Check sheet for the modelled part. Datum: model origin and axes. Units: mm. A direction names the side the tool comes from. Round coordinates to 2 decimals unless told otherwise and drop trailing zeros. Write each loop counter-clockwise with the first axis right and the second up, starting at its lowest first coordinate (ties: lowest second). Pieces come first, ordered by that corner, then holes. Notation, with made-up numbers: M -25.75,-33.75 L -17.75,-33.75 A36 ccw -17.75,2.25 Z; hole C 2,-9.75 d11. An arc over 180 degrees is marked long. Put each result on its own line as item: value.
```python
from build123d import *

# Parameters (mm, degrees)
F2_DEPTH     = 25
F3_DEPTH     = 3
F4_DEPTH     = 25
F5_R         = 4.99999
F6_T1_DEPTH  = 25
F6_T3_DEPTH  = 25
F6_T5_DEPTH  = 50
F6_T7_DEPTH  = 33.4564392374
F6_T9_DEPTH  = 50
F6_T11_DEPTH = 33.4564392374
F7_T1_DEPTH  = 16.417424305
F7_T3_DEPTH  = 20
F7_T6_ANGLE  = 89.9999999974
F7_T8_ANGLE  = 89.9999999974
F7_T10_ANGLE = 209.6926070845
F7_T12_ANGLE = 209.6926070845


# Not quite as in the source:
# - a fillet or chamfer that OpenCascade refuses, or shapes differently, is made with other operations: its cross-section is extruded or revolved along the edge and cut away or added
# - a fillet or chamfer is up to 0.001 mm smaller than in the source, because OpenCascade refuses the exact size


with BuildPart() as f2:
    # F0 (on Top) → F2 (new body)
    with BuildSketch(Plane.XY):
        Polygon((15, 36), (0, 36), (-15, 36), (-15, 22), (-15, 10), (-12, 10), (-12, 33), (0, 33), (12, 33), (12, 10), (15, 10), (15, 22), align=None)
    extrude(amount=F2_DEPTH)

    # F0 (on Top) → F3 (join)
    with BuildSketch(Plane.XY):
        Polygon((-15, 10), (-15, 22), (-37.5, 22), (-37.5, 0), (-27.5, 0), (-27.5, 10), align=None)
        Polygon((37.5, 22), (15, 22), (15, 10), (27.5, 10), (27.5, 0), (37.5, 0), align=None)
    extrude(amount=F3_DEPTH)

    # F1 (on Top) → F4 (cut)
    with BuildSketch(Plane.XY):
        with BuildLine():
            Line((35, 3.8767794613), (35, 15.8767794613))
            ThreePointArc((35, 15.8767794613), (33.5, 17.3767794613), (32, 15.8767794613))
            Line((32, 15.8767794613), (32, 3.8767794613))
            ThreePointArc((32, 3.8767794613), (33.5, 2.3767794613), (35, 3.8767794613))
        make_face()
        with BuildLine():
            ThreePointArc((-32, 15.8767794613), (-33.5, 17.3767794613), (-35, 15.8767794613))
            Line((-35, 15.8767794613), (-35, 3.8767794613))
            ThreePointArc((-35, 3.8767794613), (-33.5, 2.3767794613), (-32, 3.8767794613))
            Line((-32, 3.8767794613), (-32, 15.8767794613))
        make_face()
    extrude(amount=F4_DEPTH, mode=Mode.SUBTRACT)

    # F5 (radius 5 in the source; OpenCascade refuses exactly that, so slightly less here)
    f5_edges = [f2.edges().sort_by_distance(p)[0] for p in [
        (-37.5, 0, 1.5),
        (-27.5, 0, 1.5),
        (-37.5, 22, 1.5),
        (37.5, 22, 1.5),
        (37.5, 0, 1.5),
        (27.5, 0, 1.5),
        (27.5, 10, 1.5),
        (-27.5, 10, 1.5),
    ]]
    fillet(f5_edges, radius=F5_R)

    # F6: fillet of radius 5 on 6 edges, made by hand

    # F6_s2 → F6_t1 (join)
    with BuildSketch(Plane.XY):
        with BuildLine():
            ThreePointArc((12, 28), (10.5355339059, 31.5355339059), (7, 33))
            Line((7, 33), (12, 33))
            Line((12, 33), (12, 28))
        make_face()
    extrude(amount=F6_T1_DEPTH)

    # F6_s4 → F6_t3 (join)
    with BuildSketch(Plane.XY):
        with BuildLine():
            ThreePointArc((-7, 33), (-10.5355339059, 31.5355339059), (-12, 28))
            Line((-12, 28), (-12, 33))
            Line((-12, 33), (-7, 33))
        make_face()
    extrude(amount=F6_T3_DEPTH)

    # F6_s6 → F6_t5 (cut)
    with BuildSketch(Plane.XY.offset(-12.5)):
        with BuildLine():
            ThreePointArc((15, 31), (13.5355339059, 34.5355339059), (10, 36))
            Line((10, 36), (15, 36))
            Line((15, 36), (15, 31))
        make_face()
    extrude(amount=F6_T5_DEPTH, mode=Mode.SUBTRACT)

    # F6_s8 → F6_t7 (cut)
    with BuildSketch(Plane.XY.offset(3)):
        with BuildLine():
            ThreePointArc((12, 10), (14.1833001327, 11.8439629074), (15, 14.582575695))
            Line((15, 14.582575695), (15, 10))
            Line((15, 10), (12, 10))
        make_face()
    extrude(amount=F6_T7_DEPTH, mode=Mode.SUBTRACT)

    # F6_s10 → F6_t9 (cut)
    with BuildSketch(Plane.XY.offset(-12.5)):
        with BuildLine():
            ThreePointArc((-10, 36), (-13.5355339059, 34.5355339059), (-15, 31))
            Line((-15, 31), (-15, 36))
            Line((-15, 36), (-10, 36))
        make_face()
    extrude(amount=F6_T9_DEPTH, mode=Mode.SUBTRACT)

    # F6_s12 → F6_t11 (cut)
    with BuildSketch(Plane.XY.offset(3)):
        with BuildLine():
            ThreePointArc((-12, 10), (-14.1833001327, 11.8439629074), (-15, 14.582575695))
            Line((-15, 14.582575695), (-15, 10))
            Line((-15, 10), (-12, 10))
        make_face()
    extrude(amount=F6_T11_DEPTH, mode=Mode.SUBTRACT)

    # F7: fillet of radius 5 on 3 edges, made by hand

    # F7_s2 → F7_t1 (cut)
    with BuildSketch(Plane.XZ.offset(-31)):
        with BuildLine():
            ThreePointArc((-10, 25), (-13.5355339059, 23.5355339059), (-15, 20))
            Line((-15, 20), (-15, 25))
            Line((-15, 25), (-10, 25))
        make_face()
        with BuildLine():
            ThreePointArc((10, 25), (13.5355339059, 23.5355339059), (15, 20))
            Line((15, 20), (15, 25))
            Line((15, 25), (10, 25))
        make_face()
    extrude(amount=F7_T1_DEPTH, mode=Mode.SUBTRACT)

    # F7_s4 → F7_t3 (cut)
    with BuildSketch(Plane.YZ.offset(-10)):
        with BuildLine():
            ThreePointArc((31, 25), (34.5355339059, 23.5355339059), (36, 20))
            Line((36, 20), (36, 25))
            Line((36, 25), (31, 25))
        make_face()
    extrude(amount=F7_T3_DEPTH, mode=Mode.SUBTRACT)

    # F7_s5 → F7_t6 (revolve, cut)
    with BuildSketch(Plane.YZ.offset(9.9999999999)):
        with BuildLine():
            ThreePointArc((31, 25), (34.5355339059, 23.5355339059), (36, 20))
            Line((36, 20), (36, 25))
            Line((36, 25), (31, 25))
        make_face()
    revolve(axis=Axis((9.9999999999, 30.9999999999, 25), (0, 0, -1)), revolution_arc=F7_T6_ANGLE, mode=Mode.SUBTRACT)

    # F7_s7 → F7_t8 (revolve, cut)
    with BuildSketch(Plane.XZ.offset(-30.9999999999)):
        with BuildLine():
            ThreePointArc((-10, 25), (-13.5355339059, 23.5355339059), (-15, 20))
            Line((-15, 20), (-15, 25))
            Line((-15, 25), (-10, 25))
        make_face()
    revolve(axis=Axis((-9.9999999999, 30.9999999999, 25), (0, 0, -1)), revolution_arc=F7_T8_ANGLE, mode=Mode.SUBTRACT)

    # F7_s9 → F7_t10 (revolve, cut)
    with BuildSketch(Plane.XZ.offset(-14.5825756948)):
        with BuildLine():
            ThreePointArc((15, 20), (13.5355339059, 23.5355339059), (10, 25))
            Line((10, 25), (15, 25))
            Line((15, 25), (15, 20))
        make_face()
    revolve(axis=Axis((10.0000000002, 14.5825756948, 25), (0, 0, -1)), revolution_arc=F7_T10_ANGLE, mode=Mode.SUBTRACT)

    # F7_s11 → F7_t12 (revolve, cut)
    with BuildSketch(Plane(origin=(-8.7286422437, 15.307527957, 0), x_dir=(0, 0, 1), z_dir=(-0.4953465841, 0.8686954366, 0))):
        with BuildLine():
            ThreePointArc((25, -1.4635253083), (23.5355339059, 2.0720085977), (20, 3.5364746917))
            Line((20, 3.5364746917), (25, 3.5364746917))
            Line((25, 3.5364746917), (25, -1.4635253083))
        make_face()
    revolve(axis=Axis((-10.0000000002, 14.5825756948, 25), (0, 0, -1)), revolution_arc=F7_T12_ANGLE, mode=Mode.SUBTRACT)


solid = f2.part
```
1. Release check for a two-part mould opening along X. For faces 1 (the flat face through (-24, 22, 1)), 2 (the cylindrical face through (-33.467, 17.376, 1.479)), 3 (the flat face through (37.5, 11, 1)) record: +X half, -X half, draft (parallel to the pull), parting line (faces both ways), or undercut.
Computed values:
face 1: draft
face 2: undercut
face 3: +X half
2. Depth check by flat-ended pin: pin 1 Ø3 at (x, z) = (15.5, 16) entering from +Y; pin 2 Ø9 at (y, z) = (15.5, 11.5) entering from +X; pin 3 Ø0.9 at (x, z) = (-21.5, 1) entering from +Y; pin 4 Ø13 at (y, z) = (18.5, 6) entering from +X. Enter the tip coordinate at first touch or a pass-through.
Computed values:
pin 1: stops at y = 34
pin 2: stops at x = 15
pin 3: stops at y = 22
pin 4: stops at x = 37.5
3. Cross-section at A-A (y = 23.5). Enter the section's corners in (x, z).
Computed values:
outline: M -15,0 L -12,0 L -12,24.58 A5 ccw -15,20 Z; M 12,0 L 15,0 L 15,20 A5 ccw 12,24.58 Z
4. Scan lines: probe 1 along X at (y, z) = (27, 5); probe 2 along Z at (x, y) = (15.5, 18); probe 3 along Y at (x, z) = (-1, 12.25). Record each from-to range of solid material in increasing order.
Computed values:
probe 1: x = -15 to -12, 12 to 15
probe 2: z = 0 to 3
probe 3: y = 33 to 36
5. Cross-section at D-D (z = 15.25). Enter the section's corners in (x, y).
Computed values:
outline: M -15,14.58 A5 ccw -12,10 L -12,28 A5 cw -7,33 L 7,33 A5 cw 12,28 L 12,10 A5 ccw 15,14.58 L 15,31 A5 ccw 10,36 L -10,36 A5 ccw -15,31 Z
6. Cross-section at C-C (x = 33.5). Enter the section's corners in (y, z), then the cut area to 3 significant figures.
Computed values:
outline: M 0.1,0 L 2.38,0 L 2.38,3 L 0.1,3 Z; M 17.38,0 L 21.9,0 L 21.9,3 L 17.38,3 Z
area: 20.4 mm2
7. Cross-section at B-B (y = 7). Enter the section's corners in (x, z).
Computed values:
outline: M -37.5,0 L -35,0 L -35,3 L -37.5,3 Z; M -32,0 L -27.08,0 L -27.08,3 L -32,3 Z; M 27.08,0 L 32,0 L 32,3 L 27.08,3 Z; M 35,0 L 37.5,0 L 37.5,3 L 35,3 Z
8. Access from +Z, -Z, +X, -X, +Y, -Y to the whole of each face (thin tool, end or side, straight path). Record for faces 4 (the flat face through (32, 10, 1)), 5 (the cylindrical face through (36.07, 1.5, 1.52)), 6 (the cylindrical face through (-14.16, 11.81, 11.38)), 7 (the flat face through (-12, 19, 12)).
Computed values:
face 4: +Z, -Z
face 5: +Z, -Z, +X, -Y
face 6: +Z, -X, -Y
face 7: +Z, -Z, -Y
